```python
from build123d import *

# Parameters (mm, degrees)
BOX_W           = 33
BOX_H           = 21
BOX_DEPTH       = 10
SKETCH_W        = 2
SKETCH_H        = 21
POCKET_DEPTH    = 8
SKETCH001_W     = 9
SKETCH001_H     = 11
POCKET001_DEPTH = 1.5
SKETCH002_W     = 18
SKETCH002_H     = 13
POCKET002_DEPTH = 1.9


with BuildPart() as part:
    # Box → Box (new body)
    with BuildSketch(Plane.XY):
        with Locations((16.5, 10.5)):
            Rectangle(BOX_W, BOX_H)
    extrude(amount=BOX_DEPTH)

    # Sketch → Pocket (cut)
    with BuildSketch(Plane.XY.offset(10)):
        with Locations((1, 10.5)):
            Rectangle(SKETCH_W, SKETCH_H)
        with Locations((32, 10.5)):
            Rectangle(SKETCH_W, SKETCH_H)
    extrude(amount=-POCKET_DEPTH, mode=Mode.SUBTRACT)

    # Sketch001 → Pocket001 (cut)
    with BuildSketch(Plane.XY.offset(10)):
        with Locations((8.5, 10.5)):
            Rectangle(SKETCH001_W, SKETCH001_H)
    extrude(amount=-POCKET001_DEPTH, mode=Mode.SUBTRACT)

    # Sketch002 → Pocket002 (cut)
    with BuildSketch(Plane.XY.offset(10)):
        with Locations((22, 10.5)):
            Rectangle(SKETCH002_W, SKETCH002_H)
    extrude(amount=-POCKET002_DEPTH, mode=Mode.SUBTRACT)


solid = part.part
```
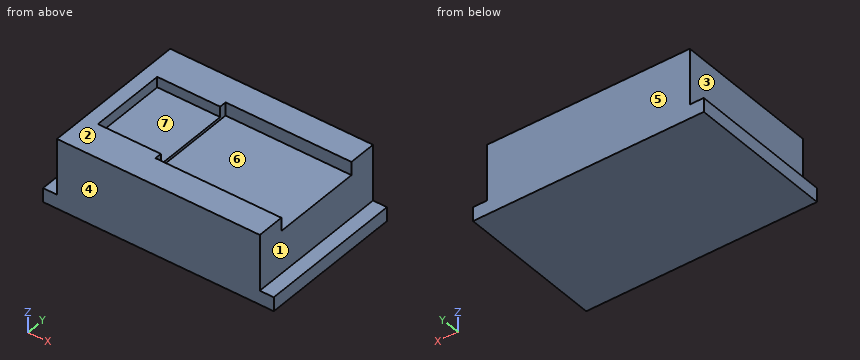
Geometry check sheet. Reference: the model listing, model coordinates, mm. Face numbers are marked on the shaded views. A direction names the side the tool comes from. Coordinates: 2 decimals unless noted, no trailing zeros. Write each loop counter-clockwise with the first axis right and the second up, starting at its lowest first coordinate (ties: lowest second). Pieces come first, ordered by that corner, then holes. Notation, with made-up numbers: M 46,60.25 L 61,60.25 A28 ccw 61,96.25 Z; hole C -20,33 d5. An arc over 180 degrees is marked long. One line per item, written item: value. Start each with the question number.
(1) Tool access check on the marked faces 1, 2 and 3. Record the directions out of +Z, -Z, +X, -X, +Y, -Y that give a thin tool (end or side, any length) a straight path to the whole face; none if there is none.
(2) Sectioned sample at C-C, the plane z = 5. Enter the section's corners in (x, y), and give its area (3 significant figures).
(3) Sectioned sample at D-D, the plane y = 14. Enter the section's corners in (x, z).
(4) Sectioned sample at A-A, the plane y = 18.5. Enter the section's corners in (x, z).
(5) Depth check by flat-ended pin: pin 1 (2 mm diameter, centred on x = 19, z = 8.5, fed in from -Y); pin 2 (0.6 mm diameter, centred on x = 32.5, y = 8, fed in from +Z); pin 3 (4.5 mm diameter, centred on x = 9, y = 9, fed in from +Z); pin 4 (6 mm diameter, centred on y = 16.5, z = 6, fed in from -X). Enter the tip coordinate at first touch or a pass-through.
(6) Scan lines: line 1 along X through (y, z) = (17.75, 7); line 2 along X through (y, z) = (15.5, 9.25); line 3 along Z through (x, y) = (22.5, 6.5). Record each from-to range of solid material in increasing order. Write a range as [from, to].
(7) Sectioned sample at B-B, the plane x = 20. Enter the section's corners in (y, z), and give its area (3 significant figures).
(8) Release check for a two-part mould opening along Y. For the marked faces 4, 5, 6 and 7 record: released by +Y, released by -Y, zero draft, split by the parting line, or undercut.
Filled sheet:
1. face 1: +Z, +X, +Y, -Y
1. face 2: +Z, +X, -X, +Y, -Y
1. face 3: +Z, -X, +Y, -Y
2. outline: M 2,0 L 31,0 L 31,21 L 2,21 Z
2. area: 609 mm²
3. outline: M 0,0 L 33,0 L 33,2 L 31,2 L 31,8.1 L 13,8.1 L 13,8.5 L 4,8.5 L 4,10 L 2,10 L 2,2 L 0,2 Z
4. outline: M 0,0 L 33,0 L 33,2 L 31,2 L 31,10 L 2,10 L 2,2 L 0,2 Z
5. pin 1: y = 0
5. pin 2: z = 2
5. pin 3: z = 8.5
5. pin 4: x = 2
6. line 1: [2, 31]
6. line 2: [2, 4]
6. line 3: [0, 8.1]
7. outline: M 0,0 L 21,0 L 21,10 L 17,10 L 17,8.1 L 4,8.1 L 4,10 L 0,10 Z
7. area: 185 mm²
8. face 4: released by -Y
8. face 5: released by +Y
8. face 6: undercut
8. face 7: undercut
